CAD build for the part. Positions are in the model's coordinates, mm. A direction names the side the tool comes from. Coordinates: 2 decimals unless noted, no trailing zeros. Order: outer loops, then holes, each group sorted by start corner. A loop starts at its lowest first (then second) coordinate and runs counter-clockwise, first axis right, second up. Notation, with made-up numbers: M 3,-16 L 57,-16 A21 cw 57,-12 Z; hole C -35.75,79.25 d9. An arc over 180 degrees is marked long. One line per item, written item: value.
from build123d import *

# Parameters (mm, degrees)
SKETCH1_W           = 60
SKETCH1_H           = 40
SKETCH1_W_2         = 20
SKETCH1_H_2         = 5
BOSS_EXTRUDE1_DEPTH = 5


with BuildPart() as part:
    # Sketch1 → Boss-Extrude1 (new body)
    with BuildSketch(Plane.XY):
        Rectangle(SKETCH1_W, SKETCH1_H)
        with Locations((-20, 22.5)):
            Rectangle(SKETCH1_W_2, SKETCH1_H_2)
        with Locations((20, -22.5)):
            Rectangle(SKETCH1_W_2, SKETCH1_H_2)
        with Locations((-20, -22.5)):
            Rectangle(SKETCH1_W_2, SKETCH1_H_2)
        with Locations((20, 22.5)):
            Rectangle(SKETCH1_W_2, SKETCH1_H_2)
    extrude(amount=BOSS_EXTRUDE1_DEPTH)


solid = part.part
Q1. Slice it at B-B (x = 1.5). List the corners of the cut face in (y, z).
Recorded:
outline: M -20,0 L 20,0 L 20,5 L -20,5 Z
Q2. Which spindle directions (+Z, -Z, +X, -X, +Y, -Y) get a long thin tool onto all of the face, cutting with end or side? Do faces 1 (the face through (-20, -25, 2)), 2 (the face through (0, -20, 2)), 3 (the face through (-10, 22, 2)). Say none if no direction does.
Recorded:
face 1: +Z, -Z, +X, -X, -Y
face 2: +Z, -Z, -Y
face 3: +Z, -Z, +Y
Q3. Drill centre line: line 1 along Y through (x, z) = (-9, 4.15). Where is it in solid material? Low to high.
Recorded:
line 1: y = -20 to 20
Q4. Pin check, flat tips, straight feed: pin 1 Ø1.5 at (x, z) = (0.5, 3) entering from +Y; pin 2 Ø1 at (x, z) = (0, 2.5) entering from -Y. Stop position of each tip, or through.
Recorded:
pin 1: stops at y = 20
pin 2: stops at y = -20
Q5. Mould opens along X. For faces 4 (the face through (20, 25, 2)), 5 (the face through (30, 0, 2)), 6 (the face through (-30, 0, 2)), 7 (the face through (10, -23, 2)) say: released by +X, released by -X, zero draft, split by the parting line, or undercut.
Recorded:
face 4: zero draft
face 5: released by +X
face 6: released by -X
face 7: undercut
Q6. Slice it at A-A (z = 1.2). List the corners of the cut face in (x, y).
Recorded:
outline: M -30,-25 L -10,-25 L -10,-20 L 10,-20 L 10,-25 L 30,-25 L 30,25 L 10,25 L 10,20 L -10,20 L -10,25 L -30,25 Z
